Model file for the job. Use its own axes, mm. A direction names the side the tool comes from. Round coordinates to 2 decimals unless told otherwise and drop trailing zeros. Order: outer loops, then holes, each group sorted by start corner. A loop starts at its lowest first (then second) coordinate and runs counter-clockwise, first axis right, second up. Notation, with made-up numbers: (60.25, -21.75) - (67.25, -21.75) arc R21 cw to (67.25, -13.75) - close; hole circle Ø9 at (10.25, -28). An arc over 180 degrees is marked (long way). Answer as CSV lines item,"result". Start each with the question number.
1. Pull direction X, two halves, no side cores. Call faces 1 (the face through (4, -4, 0)), 2 (the face through (4.261, -6.684, 5.962)), 3 (the face through (5, -3, 11)), 4 (the face through (0.602, -10.524, 5.916)): released by +X, released by -X, zero draft, split by the parting line, or undercut.
2. Band-saw the part on C-C on y = -2.5. List the corners of the cut face in (x, z).
3. Pin check, flat tip, straight feed: pin 1 Ø1 at (x, z) = (5, 3.5) entering from +Y. Stop position of the tip, or through.
4. Band-saw the part on D-D on z = 2.75. List the corners of the cut face in (x, y).
5. Band-saw the part on A-A on z = 5.75. List the corners of the cut face in (x, y), then the cut area to 3 significant figures.
6. Wall check: line 1 along Z through (x, y) = (3, -5.5); line 2 along X through (y, z) = (-2.5, 10.25); line 3 along X through (y, z) = (-2.25, 10.75). Give the ranges that are in metal, low to high. Write a range as [from, to].
7. 3-axis set-ups, long thin cutter, end or side, ignore diameter. For faces 5 (the face through (5.7, -4.2, 2.6)), 6 (the face through (6, -5, 3.25)), 7 (the face through (8.15, -2.795, 5.962)): which of +Z, -Z, +X, -X, +Y, -Y reach the whole face in a straight line?
8. Band-saw the part on B-B on x = 6.25. List the corners of the cut face in (y, z), then the cut area to 3 significant figures.
```python
from build123d import *

# Parameters (mm, degrees)
BOSS_EXTRUDE1_DEPTH = 12
BOSS_EXTRUDE2_DEPTH = 1
BOSS_EXTRUDE3_DEPTH = 1
FILLET1_R           = 1
SKETCH5_W           = 5.5
SKETCH5_H           = 5.5
CUT_EXTRUDE1_DEPTH  = 15.422205102


with BuildPart() as part:
    # Sketch1 → Boss-Extrude1 (new body)
    with BuildSketch(Plane.XY):
        Polygon((1.5, 0), (0, 0), (0, -12.02081528), (12.02081528, 0), (9.899494937, 0), (8.399494937, -1.5), (1.5, -8.399494937), (1.5, -1.5), align=None)
    extrude(amount=BOSS_EXTRUDE1_DEPTH)

    # Sketch2 → Boss-Extrude2 (add)
    with BuildSketch(Plane.XY.offset(12)):
        Polygon((0, 0), (12.02081528, 0), (0, -12.02081528), align=None)
    extrude(amount=-BOSS_EXTRUDE2_DEPTH)

    # Sketch3 → Boss-Extrude3 (add)
    with BuildSketch(Plane(origin=(0, 0, 0), x_dir=(-1, 0, 0), z_dir=(0, 0, -1))):
        Polygon((-12.02081528, 0), (0, 0), (0, -12.02081528), align=None)
    extrude(amount=-BOSS_EXTRUDE3_DEPTH)

    # Fillet1
    # the kernel refuses this fillet: 1 mm, written as the material it takes off along each edge
    with BuildSketch(Plane(origin=(0, -12.02081528, -6.035533906), x_dir=(0, 1, 0), z_dir=(0, 0, 1)), Plane(origin=(12.02081528, 0, 18.035533906), x_dir=(-1, 0, 0), z_dir=(0, 0, -1))) as fillet1_piece_1:
        with BuildLine():
            CenterArc((FILLET1_R * 2.41421356237, -FILLET1_R), FILLET1_R, 90, 135)
            Line((FILLET1_R * 1.70710678119, -FILLET1_R * 1.70710678119), (0, 0))
            Line((0, 0), (FILLET1_R * 2.41421356237, 0))
        make_face()
    extrude(amount=24.071067812, mode=Mode.SUBTRACT)

    # Sketch5 → Cut-Extrude1 (cut, through all)
    with BuildSketch(Plane(origin=(4.949747468, -4.949747468, 0), x_dir=(0, 0, 1), z_dir=(-0.7071067811865476, 0.7071067811865475, 0))):
        with Locations((6, 1.036566092)):
            Rectangle(SKETCH5_W, SKETCH5_H)
    extrude(amount=-CUT_EXTRUDE1_DEPTH, mode=Mode.SUBTRACT)


solid = part.part
```
Reply:
1,face 1,"zero draft"
1,face 2,"released by +X"
1,face 3,"undercut"
1,face 4,"split by the parting line"
2,outline,"(0, 0) - (9.52, 0) - (9.52, 12) - (0, 12) - close; hole (1.5, 1) - (7.4, 1) - (7.4, 3.25) - (7.86, 3.25) - (7.86, 8.75) - (7.4, 8.75) - (7.4, 11) - (1.5, 11) - close"
3,pin 1,"stops at y = -4.47"
4,outline,"(0, -9.61) arc R1 ccw to (1.71, -10.31) - (10.31, -1.71) arc R1 ccw to (9.87, -0.03) - (1.5, -8.4) - (1.5, 0) - (0, 0) - close"
5,outline,"(0, -9.61) arc R1 ccw to (1.71, -10.31) - (4.8, -7.22) - (3.74, -6.16) - (1.5, -8.4) - (1.5, 0) - (0, 0) - close; (7.63, -2.27) - (8.69, -3.33) - (10.31, -1.71) arc R1 ccw to (9.87, -0.03) - close"
5,area,"26.3 mm2"
6,line 1,"z = [0, 1], [11, 12]"
6,line 2,"x = [0, 1.5], [7.4, 9.52]"
6,line 3,"x = [0, 1.5], [7.65, 9.77]"
7,face 5,"+Y"
7,face 6,"none"
7,face 7,"-Y"
8,outline,"(-5.77, 0) - (0, 0) - (0, 1) - (-3.65, 1) - (-3.65, 3.25) - (-5.77, 3.25) - close; (-5.77, 8.75) - (-3.65, 8.75) - (-3.65, 11) - (0, 11) - (0, 12) - (-5.77, 12) - close"
8,area,"21.1 mm2"
